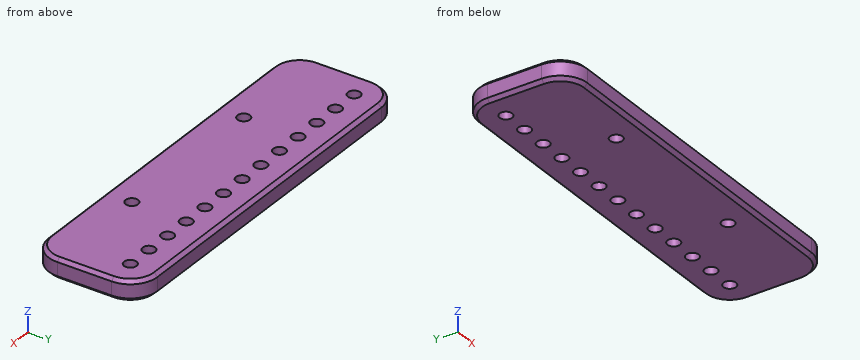
```python
from build123d import *

# Parameters (mm, degrees)
SKETCH1_W           = 177.8
SKETCH1_H           = 50.8
SKETCH1_R           = 2.921
BOSS_EXTRUDE1_DEPTH = 9.525
FILLET1_R           = 12.7
CHAMFER1_SIZE       = 1.5875


with BuildPart() as part:
    # Sketch1 → Boss-Extrude1 (new body)
    with BuildSketch(Plane.XY):
        with Locations((88.9, 25.4)):
            Rectangle(SKETCH1_W, SKETCH1_H)
        with Locations(Location((50.8, 12.7, 0), (0, 0, 180))):
            Circle(SKETCH1_R, mode=Mode.SUBTRACT)
        with Locations(Location((127, 12.7, 0), (0, 0, 180))):
            Circle(SKETCH1_R, mode=Mode.SUBTRACT)
        with Locations(Location((12.7, 38.1, 0), (0, 0, 180))):
            Circle(SKETCH1_R, mode=Mode.SUBTRACT)
        with Locations(Location((25.4, 38.1, 0), (0, 0, 180))):
            Circle(SKETCH1_R, mode=Mode.SUBTRACT)
        with Locations(Location((38.1, 38.1, 0), (0, 0, 180))):
            Circle(SKETCH1_R, mode=Mode.SUBTRACT)
        with Locations(Location((50.8, 38.1, 0), (0, 0, 180))):
            Circle(SKETCH1_R, mode=Mode.SUBTRACT)
        with Locations(Location((63.5, 38.1, 0), (0, 0, 180))):
            Circle(SKETCH1_R, mode=Mode.SUBTRACT)
        with Locations(Location((76.2, 38.1, 0), (0, 0, 180))):
            Circle(SKETCH1_R, mode=Mode.SUBTRACT)
        with Locations(Location((88.9, 38.1, 0), (0, 0, 180))):
            Circle(SKETCH1_R, mode=Mode.SUBTRACT)
        with Locations(Location((101.6, 38.1, 0), (0, 0, 180))):
            Circle(SKETCH1_R, mode=Mode.SUBTRACT)
        with Locations(Location((114.3, 38.1, 0), (0, 0, 180))):
            Circle(SKETCH1_R, mode=Mode.SUBTRACT)
        with Locations(Location((127, 38.1, 0), (0, 0, 180))):
            Circle(SKETCH1_R, mode=Mode.SUBTRACT)
        with Locations(Location((139.7, 38.1, 0), (0, 0, 180))):
            Circle(SKETCH1_R, mode=Mode.SUBTRACT)
        with Locations(Location((152.4, 38.1, 0), (0, 0, 180))):
            Circle(SKETCH1_R, mode=Mode.SUBTRACT)
        with Locations(Location((165.1, 38.1, 0), (0, 0, 180))):
            Circle(SKETCH1_R, mode=Mode.SUBTRACT)
    extrude(amount=BOSS_EXTRUDE1_DEPTH)

    # Fillet1
    fillet1_edges = [part.edges().sort_by_distance(p)[0] for p in [
        (0, 50.8, 4.7625),
        (177.8, 50.8, 4.7625),
        (177.8, 0, 4.7625),
        (0, 0, 4.7625),
    ]]
    fillet(fillet1_edges, radius=FILLET1_R)

    # Chamfer1
    chamfer1_edges = [part.edges().sort_by_distance(p)[0] for p in [
        (88.9, 0, 0),
        (88.9, 0, 9.525),
        (0, 25.4, 0),
        (88.9, 50.8, 0),
        (177.8, 25.4, 0),
        (174.080256121, 47.080256121, 0),
        (174.080256121, 3.719743879, 0),
        (3.719743879, 47.080256121, 0),
        (3.719743879, 3.719743879, 0),
        (0, 25.4, 9.525),
        (177.8, 25.4, 9.525),
        (88.9, 50.8, 9.525),
        (174.080256121, 47.080256121, 9.525),
        (174.080256121, 3.719743879, 9.525),
        (3.719743879, 47.080256121, 9.525),
        (3.719743879, 3.719743879, 9.525),
    ]]
    chamfer(chamfer1_edges, length=CHAMFER1_SIZE)


solid = part.part
```
Check sheet for the modelled part. Datum: model origin and axes. Units: mm. Round coordinates to 2 decimals unless told otherwise and drop trailing zeros. Write each loop counter-clockwise with the first axis right and the second up, starting at its lowest first coordinate (ties: lowest second). Pieces come first, ordered by that corner, then holes. Notation, with made-up numbers: M 52.25,45.5 L 104.25,45.5 A29 cw 104.25,68.5 Z; hole C 70.25,-24 d6. An arc over 180 degrees is marked long. Write item = value, one per line. Start each with the question number.
1. Section check B-B, the plane x = 101.6. Record the cut outline in (y, z) (1 decimal).
2. Gauge pin test, flat ends, axial feed: pin 1 (7.5 mm diameter, centred on x = 38.1, y = 38.1, fed in from -Z); pin 2 (1 mm diameter, centred on y = 7.5, z = 3.5, fed in from +X); pin 3 (4.5 mm diameter, centred on x = 50.8, y = 38.1, fed in from -Z); pin 4 (1 mm diameter, centred on y = 42, z = 4, fed in from -X). Record the tip position at first contact, or that the pin passes through.
3. Scan lines: line 1 (Y direction, x = 139.7, z = 7); line 2 (Y direction, x = 48.5, z = 7.75); line 3 (Y direction, x = 151, z = 1.5). Record each from-to range of solid material in increasing order. Write a range as [from, to].
4. Section check A-A, the plane x = 127. Record the cut outline in (y, z) (1 decimal), then the cut area to 3 significant figures.
Results found:
q1.outline = M 0,1.6 L 1.6,0 L 35.2,0 L 35.2,9.5 L 1.6,9.5 L 0,7.9 Z; M 41,0 L 49.2,0 L 50.8,1.6 L 50.8,7.9 L 49.2,9.5 L 41,9.5 Z
q2.pin_1 = 0
q2.pin_2 = 176.9
q2.pin_3 = through
q2.pin_4 = 0.46
q3.line_1 = [0, 35.18], [41.02, 50.8]
q3.line_2 = [0, 10.9], [14.5, 36.3], [39.9, 50.8]
q3.line_3 = [0.09, 35.54], [40.66, 50.71]
q4.outline = M 0,1.6 L 1.6,0 L 9.8,0 L 9.8,9.5 L 1.6,9.5 L 0,7.9 Z; M 15.6,0 L 35.2,0 L 35.2,9.5 L 15.6,9.5 Z; M 41,0 L 49.2,0 L 50.8,1.6 L 50.8,7.9 L 49.2,9.5 L 41,9.5 Z
q4.area = 368 mm^2
